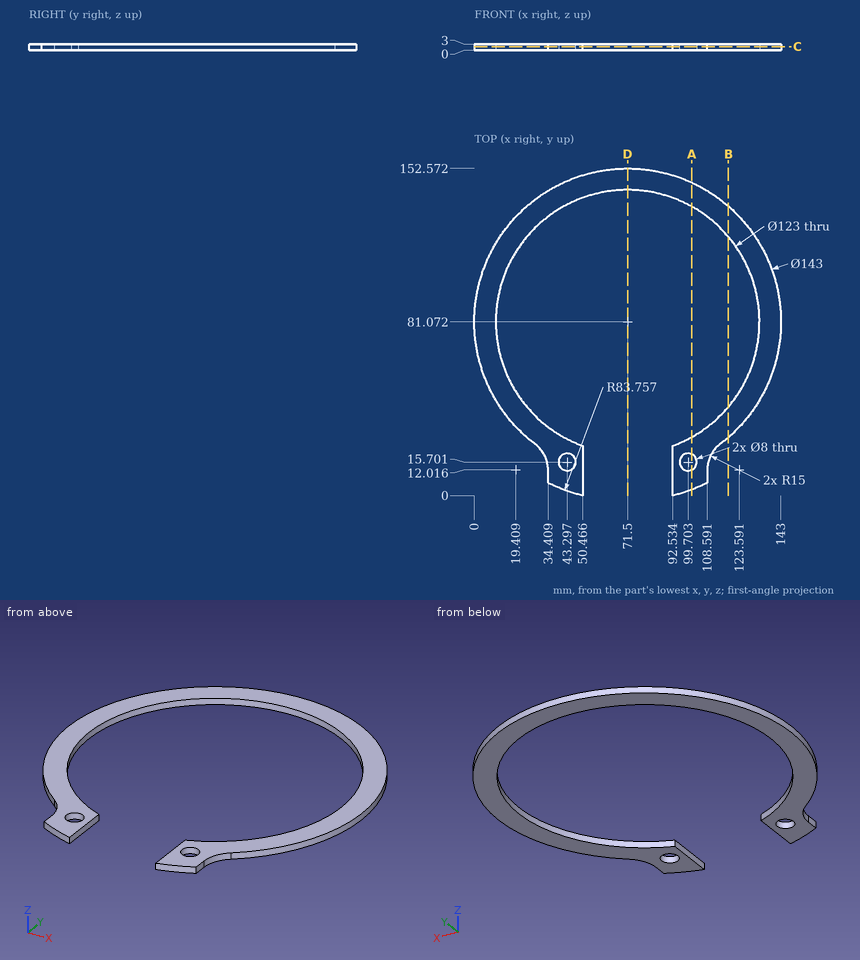
Geometry check sheet. Reference: drawing and pictorial views, mm from the part's lowest x, y, z. Coordinates: 2 decimals unless noted, no trailing zeros. Order: outer loops, then holes, each group sorted by start corner. A loop starts at its lowest first (then second) coordinate and runs counter-clockwise, first axis right, second up. Notation, with made-up numbers: M 56.25,29 L 97.25,29 A18 cw 97.25,47 Z; hole C -17.75,-37.75 d11. An arc over 180 degrees is marked long. Write each question's results on one line, items separated by ' | '. Start each with the question number.
1. Material ranges on probe 1 along X at (y, z) = (9, 1.5) (1 decimal); probe 2 along X at (y, z) = (79.5, 1.1); probe 3 along Y at (x, z) = (46.5, 2.1) (1 decimal), recorded low to high.
2. Cross-section at C-C on z = 1.75. Record the cut outline in (x, y) (1 decimal).
3. Cross-section at B-B on x = 118.5. Record the cut outline in (y, z) (1 decimal).
4. Cross-section at A-A on x = 101.5. Record the cut outline in (y, z) (1 decimal).
5. Cross-section at D-D on x = 71.5. Record the cut outline in (y, z).
6. Go/stop test with flat-tipped pins: P1, Ø1.5, axis at x = 29.5, z = 1, coming from the -Y side; P2, Ø0.9, axis at y = 10, z = 1.5, coming from the -X side; P3, Ø13, axis at x = 43.3, y = 15.7, coming from the +Z side; P4, Ø1.5, axis at y = 70, z = 1, coming from the -X side. Record where each tip stops, or that it passes through.
Checks:
1) probe 1: x = 34.4 to 50.5, 92.5 to 108.6 | probe 2: x = 0.02 to 10.02, 132.98 to 142.98 | probe 3: y = 1.1 to 13.3, 18.1 to 24.9, 137.3 to 148.1
2) outline: M 28.4,24 A15 cw 34.4,12 L 34.4,6 A83.8 ccw 50.5,0 L 50.5,23.3 A61.5 cw long 92.5,23.3 L 92.5,0 A83.8 ccw 108.6,6 L 108.6,12 A15 cw 114.6,24 A71.5 ccw long Z; hole C 43.3,15.7 d8; hole C 99.7,15.7 d8
3) outline: M 27.2,0 L 41.4,0 L 41.4,3 L 27.2,3 Z; M 120.7,0 L 135,0 L 135,3 L 120.7,3 Z
4) outline: M 2.9,0 L 12.1,0 L 12.1,3 L 2.9,3 Z; M 19.3,0 L 27.4,0 L 27.4,3 L 19.3,3 Z; M 134.8,0 L 146,0 L 146,3 L 134.8,3 Z
5) outline: M 142.57,0 L 152.57,0 L 152.57,3 L 142.57,3 Z
6) P1: stops at y = 22.38 | P2: stops at x = 34.41 | P3: stops at z = 3 | P4: stops at x = 0.75
